The listing builds one solid part. Answer for the finished solid, in the listing's coordinates (mm). A direction names the side the tool comes from. Coordinates: 2 decimals unless noted, no trailing zeros. Order: outer loops, then holes, each group sorted by start corner. A loop starts at its lowest first (then second) coordinate and runs counter-clockwise, first axis right, second up. Notation, with made-up numbers: (-31, -29) -> (-25, -29) arc R19 ccw to (-25, -18) -> close; hole circle Ø9 at (6, 54). An arc over 180 degrees is marked (long way). Answer in a Markdown table with one row per item.
```python
from build123d import *

# Parameters (mm, degrees)
SKETCH1_R           = 12.5
BOSS_EXTRUDE1_DEPTH = 6
CUT_EXTRUDE1_DEPTH  = 19.668154703
SKETCH3_R           = 1.5
CUT_EXTRUDE2_DEPTH  = 19.668154703


with BuildPart() as part:
    # Sketch1 → Boss-Extrude1 (new body)
    with BuildSketch(Plane(origin=(0, 0, 0), x_dir=(1, 0, 0), z_dir=(0, 1, 0))):
        with Locations(Location((0, 0, 0), (0, 0, 270))):
            Circle(SKETCH1_R)
    extrude(amount=BOSS_EXTRUDE1_DEPTH)

    # Sketch2 → Cut-Extrude1 (cut, through all)
    with BuildSketch(Plane(origin=(0, 6, 0), x_dir=(1, 0, 0), z_dir=(0, 1, 0))):
        with BuildLine():
            Line((-2.5, -1.5), (-2.5, 1.5))
            ThreePointArc((-2.5, 1.5), (0, 4), (2.5, 1.5))
            Line((2.5, 1.5), (2.5, -1.5))
            ThreePointArc((2.5, -1.5), (0, -4), (-2.5, -1.5))
        make_face()
    extrude(amount=-CUT_EXTRUDE1_DEPTH, mode=Mode.SUBTRACT)

    # Sketch3 → Cut-Extrude2 (cut, through all)
    with BuildSketch(Plane(origin=(0, 6, 0), x_dir=(1, 0, 0), z_dir=(0, 1, 0))):
        with Locations(Location((-9, 0, 0), (0, 0, 270))):
            Circle(SKETCH3_R)
        with Locations(Location((9, 0, 0), (0, 0, 90))):
            Circle(SKETCH3_R)
    extrude(amount=-CUT_EXTRUDE2_DEPTH, mode=Mode.SUBTRACT)


solid = part.part
```
(1) A cutting plane is placed at B-B, the plane y = 2.15. Determine the outline of the cut face in (x, z).
Check values:
| item | result |
|---|---|
| outline | circle Ø25 at (0, 0); hole circle Ø3 at (-9, 0); hole (-2.5, -1.5) arc R2.5 ccw to (2.5, -1.5) -> (2.5, 1.5) arc R2.5 ccw to (-2.5, 1.5) -> close; hole circle Ø3 at (9, 0) |
(2) Which of the six approach directions +Z, -Z, +X, -X, +Y, -Y give full straight-line access (tool end or side, diameter ignored) to faces 1 (the flat face through (2.5, 3, 0)), 2 (the flat face through (-3, 0, 0))?
Check values:
| item | result |
|---|---|
| face 1 | +Y, -Y |
| face 2 | +Z, -Z, +X, -X, -Y |
(3) For a pull along Z with two mould halves and no side action, classify faces 3 (the cylindrical face through (3.755, 2.958, 11.923)), 4 (the flat face through (-3, 6, 0)), 5 (the cylindrical face through (0, 3, 4)) as released by +Z, released by -Z, zero draft, split by the parting line, or undercut.
Check values:
| item | result |
|---|---|
| face 3 | split by the parting line |
| face 4 | zero draft |
| face 5 | undercut |
(4) A cutting plane is placed at A-A, the plane z = 0. Determine the outline of the cut face in (x, y), then the cut area to 3 significant figures.
Check values:
| item | result |
|---|---|
| outline | (-12.5, 0) -> (-10.5, 0) -> (-10.5, 6) -> (-12.5, 6) -> close; (-7.5, 0) -> (-2.5, 0) -> (-2.5, 6) -> (-7.5, 6) -> close; (2.5, 0) -> (7.5, 0) -> (7.5, 6) -> (2.5, 6) -> close; (10.5, 0) -> (12.5, 0) -> (12.5, 6) -> (10.5, 6) -> close |
| area | 84.0 mm² |
(5) A cutting plane is placed at D-D, the plane x = -0.5. Determine the outline of the cut face in (y, z), then the cut area to 3 significant figures.
Check values:
| item | result |
|---|---|
| outline | (0, -12.49) -> (6, -12.49) -> (6, -3.95) -> (0, -3.95) -> close; (0, 3.95) -> (6, 3.95) -> (6, 12.49) -> (0, 12.49) -> close |
| area | 102 mm² |
(6) Find the intervals of material crossed by line 1 along X through (y, z) = (1.4, 0); line 2 along Z through (x, y) = (9, 3.75); line 3 along X through (y, z) = (2.85, -3), in increasing order. Write a range as from..to.
Check values:
| item | result |
|---|---|
| line 1 | -12.5..-10.5, -7.5..-2.5, 2.5..7.5, 10.5..12.5 |
| line 2 | -8.67..-1.5, 1.5..8.67 |
| line 3 | -12.13..-2, 2..12.13 |
(7) A cutting plane is placed at C-C, the plane x = 9. Determine the outline of the cut face in (y, z).
Check values:
| item | result |
|---|---|
| outline | (0, -8.67) -> (6, -8.67) -> (6, -1.5) -> (0, -1.5) -> close; (0, 1.5) -> (6, 1.5) -> (6, 8.67) -> (0, 8.67) -> close |
(8) Flat-ended cylindrical pins translate along their axes: pin 1 (1 mm diameter, centred on y = 2.5, z = 8.5, fed in from +X); pin 2 (3.5 mm diameter, centred on y = 3, z = 0.5, fed in from -X); pin 3 (3 mm diameter, centred on x = -3, y = 5, fed in from +Z); pin 4 (1 mm diameter, centred on y = 3.5, z = 5, fed in from -X). Find the tip coordinate at first contact, or state that the pin passes through.
Check values:
| item | result |
|---|---|
| pin 1 | x = 9.6 |
| pin 2 | x = -12.5 |
| pin 3 | z = 12.41 |
| pin 4 | x = -11.66 |
